Verification items for the finished model (mm, model axes). Coordinates: 2 decimals unless noted, no trailing zeros. Order: outer loops, then holes, each group sorted by start corner. A loop starts at its lowest first (then second) coordinate and runs counter-clockwise, first axis right, second up. Notation, with made-up numbers: (15.25, -23.75) -> (33.25, -23.75) arc R31 ccw to (33.25, 3.25) -> close; hole circle Ø5 at (85, 64). An arc over 180 degrees is marked (long way). Answer as CSV lines item,"result".
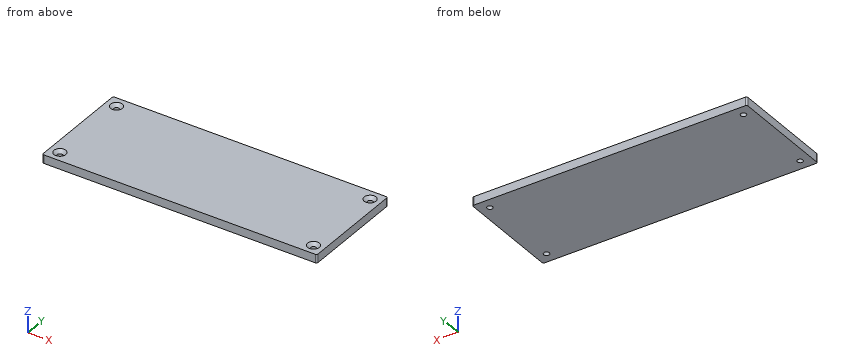
```python
from build123d import *

# Parameters (mm, degrees)
F0_W           = 260
F0_H           = 100
F1_DEPTH       = 8
F2_D           = 5.25
F2_CSINK_D     = 11.2
F2_CSINK_ANGLE = 90
F3_R           = 1.5


# Not quite as in the source:
# - a feature names something its author has since deleted; it is built from what else it names


with BuildPart() as f1:
    # F0 (on Top) → F1 (new body)
    with BuildSketch(Plane.XY):
        with Locations((-130, 50)):
            Rectangle(F0_W, F0_H)
    extrude(amount=-F1_DEPTH)

    # F2 (through all)
    with Locations(Plane.XY):
        with Locations((-250, 10), (-10, 10), (-10, 90), (-250, 90)):
            CounterSinkHole(F2_D / 2, F2_CSINK_D / 2, counter_sink_angle=F2_CSINK_ANGLE)

    # F3
    f3_edges = [f1.edges().sort_by_distance(p)[0] for p in [
        (0, 0, -4),
        (0, 100, -4),
        (-260, 0, -4),
        (-260, 100, -4),
    ]]
    fillet(f3_edges, radius=F3_R)


solid = f1.part
```
Item 1: Thickness scan on line 1 (Y direction, x = -10, z = -4.8) (3 decimals); line 2 (X direction, y = 10, z = -4.7) (3 decimals). Record the ranges inside material, lowest first.
Answer list:
line 1,"0 to 7.375, 12.625 to 87.375, 92.625 to 100"
line 2,"-260 to -252.625, -247.375 to -12.625, -7.375 to 0"
Item 2: Section check A-A, the plane y = 10. Record the boundary of the cut face in (x, z) (3 decimals), plus the area to 3 significant figures.
Answer list:
outline,"(-260, -8) -> (-252.625, -8) -> (-252.625, -2.975) -> (-255.6, 0) -> (-260, 0) -> close; (-247.375, -8) -> (-12.625, -8) -> (-12.625, -2.975) -> (-15.6, 0) -> (-244.4, 0) -> (-247.375, -2.975) -> close; (-7.375, -8) -> (0, -8) -> (0, 0) -> (-4.4, 0) -> (-7.375, -2.975) -> close"
area,"1,980 mm2"
Item 3: Section check B-B, the plane x = -250. Record the boundary of the cut face in (y, z) (3 decimals), plus the area to 3 significant figures.
Answer list:
outline,"(0, -8) -> (7.375, -8) -> (7.375, -2.975) -> (4.4, 0) -> (0, 0) -> close; (12.625, -8) -> (87.375, -8) -> (87.375, -2.975) -> (84.4, 0) -> (15.6, 0) -> (12.625, -2.975) -> close; (92.625, -8) -> (100, -8) -> (100, 0) -> (95.6, 0) -> (92.625, -2.975) -> close"
area,"698 mm2"
Item 4: Depth check by flat-ended pin: pin 1 Ø7 at (x, y) = (-10, 90) entering from +Z; pin 2 Ø6 at (x, y) = (-250, 90) entering from +Z. Enter the tip coordinate at first touch or a pass-through.
Answer list:
pin 1,"z = -2.1"
pin 2,"z = -2.6"
